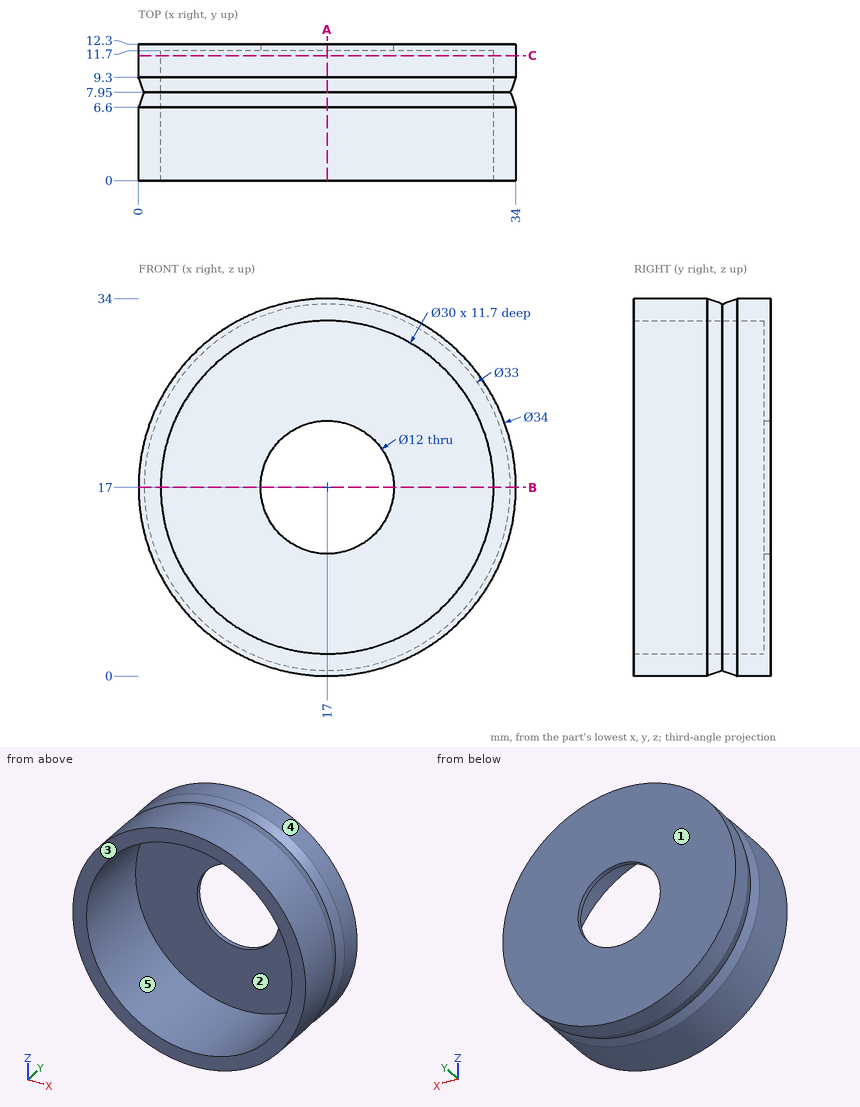
Here's the drawing with two shaded views (mm, measured from the low corner). I have some questions. A direction names the side the tool comes from. Coordinates: 2 decimals unless noted, no trailing zeros. Write each loop counter-clockwise with the first axis right and the second up, starting at its lowest first coordinate (ties: lowest second). Pieces come first, ordered by that corner, then holes. Notation, with made-up numbers: M 53,23 L 104,23 A9 ccw 104,33 Z; hole C 34.5,0.25 d5. An arc over 180 degrees is marked long. Answer as CSV lines item,"result". Start each with the question number.
1) I want a section at B-B, the plane z = 17. Please give me the cut outline in (x, y).
2) We'd pull the mould along X, two halves only. Please class the marked faces 3, 4 and 5: +X half, -X half, draft (parallel to the pull), parting line (faces both ways), or undercut.
3) I want a section at A-A, the plane x = 17. Please give me the cut outline in (y, z).
4) For P1, Ø6, axis at x = 7, y = 6.5, coming from the -Z side; P2, Ø4, axis at x = 4, y = 4.5, coming from the +Z side; P3, Ø3, axis at x = 8.5, z = 18.5, coming from the -Y side, each with a flat end and sliding along its axis, tell me the tip position at first contact or that it passes through.
5) I want a section at C-C, the plane y = 11.25. Please give me the cut outline in (x, z), and give its area (3 significant figures).
6) Please list where these lines run through material, in increasing order: line 1 (Z direction, x = 17, y = 5.5); line 2 (Z direction, x = 17, y = 12); line 3 (Y direction, x = 13.5, z = 2.5). Write a range as from..to.
7) For the marked faces 1 and 2, which set-ups out of +Z, -Z, +X, -X, +Y, -Y let a thin tool reach every point of the face, with its end or its side?
Data:
1,outline,"M 0,0 L 2,0 L 2,11.7 L 11,11.7 L 11,12.3 L 0,12.3 L 0,9.3 L 0.5,7.95 L 0,6.6 Z; M 23,11.7 L 32,11.7 L 32,0 L 34,0 L 34,6.6 L 33.5,7.95 L 34,9.3 L 34,12.3 L 23,12.3 Z"
2,face 3,"draft"
2,face 4,"parting line"
2,face 5,"undercut"
3,outline,"M 0,0 L 6.6,0 L 7.95,0.5 L 9.3,0 L 12.3,0 L 12.3,11 L 11.7,11 L 11.7,2 L 0,2 Z; M 0,32 L 11.7,32 L 11.7,23 L 12.3,23 L 12.3,34 L 9.3,34 L 7.95,33.5 L 6.6,34 L 0,34 Z"
4,P1,"stops at z = 1.51"
4,P2,"stops at z = 29.96"
4,P3,"stops at y = 11.7"
5,outline,"C 17,17 d34; hole C 17,17 d30"
5,area,"201 mm^2"
6,line 1,"z = 0..2, 32..34"
6,line 2,"z = 0..11, 23..34"
6,line 3,"y = 11.7..12.3"
7,face 1,"+Z, -Z, +X, -X, +Y"
7,face 2,"-Y"
